Could you check a few things on this model? Use its own coordinates, in mm. Face numbers are marked on the shaded views. A direction names the side the tool comes from. Round coordinates to 2 decimals unless told otherwise and drop trailing zeros. Loops run counter-clockwise (first coordinate to the right, second up) from the corner with the lowest first, then second, coordinate; pieces in that order, holes last. Notation, with made-up numbers: (-3.5, 14.25) - (45.5, 14.25) arc R23 cw to (45.5, 39.25) - close; hole circle Ø10 at (41.25, 4). An arc over 180 degrees is marked (long way). Answer as CSV lines item,"result". Start each with the question number.
1) Suppose I cut it at A-A, the plane z = 0. Write out the boundary of the cut face in (x, y).
2) Suppose I cut it at D-D, the plane y = 7.75. Write out the boundary of the cut face in (x, z).
3) Suppose I cut it at B-B, the plane y = 2.5. Write out the boundary of the cut face in (x, z), then the cut area to 3 significant figures.
4) We'd pull the mould along X, two halves only. Please class the marked faces 3, 4, 5 and 6: pulls with the +X half, pulls with the -X half, needs draft (parallel to the pull), parting line crosses it, or undercut.
5) I'm going to push flat-ended pins straight in: pin 1 Ø2 at (x, z) = (-10.5, -1) entering from +Y; pin 2 Ø3 at (x, y) = (8, 4) entering from -Z; pin 3 Ø4 at (x, y) = (-15, 1.5) entering from -Z; pin 4 Ø1.8 at (y, z) = (0.5, 0.5) entering from -X. Where does each tip first touch, or does it pass through?
6) Which directions (+Z, -Z, +X, -X, +Y, -Y) give clear straight access to the entire face, cutting with the end or side of a thin tool? Please do the marked faces 1 and 2.
7) Suppose I cut it at C-C, the plane x = 8. Write out the boundary of the cut face in (y, z), then the cut area to 3 significant figures.
8) Please list where these lines run through material, in increasing order: line 1 along X through (y, z) = (-1.75, -0.85); line 2 along Z through (x, y) = (-8, 0); line 3 along X through (y, z) = (1.75, -0.3).
```python
from build123d import *

# Parameters (mm, degrees)
SKETCH1_R           = 1.5
BOSS_EXTRUDE1_DEPTH = 10.5
SKETCH2_R           = 2.95
BOSS_EXTRUDE2_DEPTH = 0.9
SWEEP1_PROFILE_R    = 0.85


with BuildPart() as part:
    # Sketch1 → Boss-Extrude1 (new body)
    with BuildSketch(Plane(origin=(0, 0, 0), x_dir=(0, 0, -1), z_dir=(1, 0, 0))):
        with Locations(Location((0, 0, 0), (0, 0, 180))):
            Circle(SKETCH1_R)
    extrude(amount=BOSS_EXTRUDE1_DEPTH)

    # Sketch8 → Revolve1 (revolve)
    with BuildSketch(Plane(origin=(10.5, 0, 0), x_dir=(0, 0, -1), z_dir=(1, 0, 0))):
        with BuildLine():
            Line((1.5, 0), (-1.5, 0))
            ThreePointArc((-1.5, 0), (0, 1.5), (1.5, 0))
        make_face()
    revolve(axis=Axis((10.5, 0, -1.5), (0, 0, 1)))

    # Sketch2 → Boss-Extrude2 (add)
    with BuildSketch(Plane.ZY):
        Circle(SKETCH2_R)
    extrude(amount=BOSS_EXTRUDE2_DEPTH)

    # Sweep1: sweep along a path in Sketch3
    with BuildLine(Plane.XY) as sweep1_path:
        Line((-0.9, 0), (-15.9, 0))
        ThreePointArc((-15.9, 0), (-16.960660172, 0.439339828), (-17.4, 1.5))
        Line((-17.4, 1.5), (-17.4, 9.5))
    # Sweep1 profile (on start of the path) → Sweep1 (sweep)
    with BuildSketch(Plane(origin=(-0.9, 0, 0), x_dir=(0, -1, 0), z_dir=(-1, 0, 0))):
        Circle(SWEEP1_PROFILE_R)
    sweep(path=sweep1_path.line)


solid = part.part
```
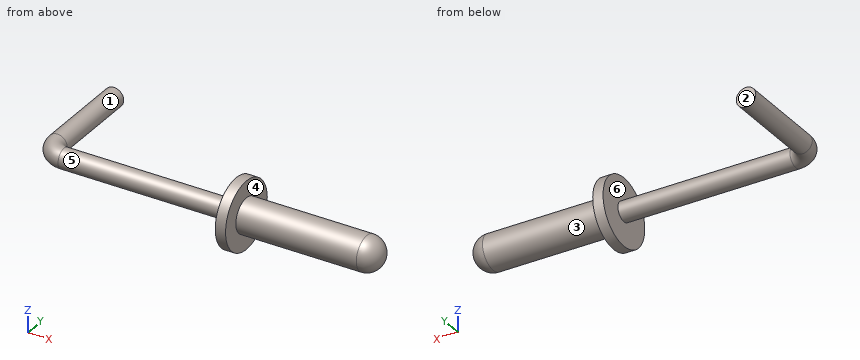
Filled sheet:
1,outline,"(-18.25, 1.5) arc R2.35 ccw to (-15.9, -0.85) - (-0.9, -0.85) - (-0.9, -2.95) - (0, -2.95) - (0, -1.5) - (10.5, -1.5) arc R1.5 ccw to (10.5, 1.5) - (0, 1.5) - (0, 2.95) - (-0.9, 2.95) - (-0.9, 0.85) - (-15.9, 0.85) arc R0.65 cw to (-16.55, 1.5) - (-16.55, 9.5) - (-18.25, 9.5) - close"
2,outline,"circle Ø1.7 at (-17.4, 0)"
3,outline,"circle Ø1.7 at (-17.4, 0); (-0.9, -1.57) - (0, -1.57) - (0, 1.57) - (-0.9, 1.57) - close"
3,area,"5.09 mm²"
4,face 3,"needs draft"
4,face 4,"pulls with the +X half"
4,face 5,"undercut"
4,face 6,"undercut"
5,pin 1,"y = 0.85"
5,pin 2,"through"
5,pin 3,"z = -0.85"
5,pin 4,"x = -18.24"
6,face 1,"+Y"
6,face 2,"+Z, -Z, +X, -X, +Y"
7,outline,"circle Ø3 at (0, 0)"
7,area,"7.07 mm²"
8,line 1,"-0.9 to 0"
8,line 2,"-0.85 to 0.85"
8,line 3,"-18.2 to -16.6, -0.9 to 0"
